```python
from build123d import *

# Parameters (mm, degrees)
PAD001_DEPTH = 12
SKETCH_W     = 24
SKETCH_H     = 12
SKETCH_R     = 1.3
PAD_DEPTH    = 2
FILLET_R     = 3
FILLET001_R  = 0.5


with BuildPart() as pad001:
    # Sketch001 → Pad001 (new body, symmetric)
    with BuildSketch(Plane.YZ):
        Polygon((0, 0), (0, 6), (2, 6), (2, 8), (0, 8), (0, 9), (7, 9), (7, 0), align=None)
    extrude(amount=PAD001_DEPTH, both=True)


with BuildPart() as fillet001:
    # Sketch → Pad (new body)
    with BuildSketch(Plane.XY):
        with Locations((0, 6)):
            Rectangle(SKETCH_W, SKETCH_H)
        with Locations((-8, 9.5)):
            Circle(SKETCH_R, mode=Mode.SUBTRACT)
        with Locations((0, 9.5)):
            Circle(SKETCH_R, mode=Mode.SUBTRACT)
        with Locations((8, 9.5)):
            Circle(SKETCH_R, mode=Mode.SUBTRACT)
    extrude(amount=-PAD_DEPTH)

    # Fusion: union Pad001
    add(pad001.part)

    # Fillet
    fillet_edges = [fillet001.edges().sort_by_distance(p)[0] for p in [
        (0, 7, 9),
    ]]
    fillet(fillet_edges, radius=FILLET_R)

    # Fillet001
    fillet001_edges = [fillet001.edges().sort_by_distance(p)[0] for p in [
        (0, 7, 0),
    ]]
    fillet(fillet001_edges, radius=FILLET001_R)


solid = fillet001.part
```
Here's how the part is built. I have some questions about the finished solid (model axes, mm). A direction names the side the tool comes from. Give positions to 0.01 mm unless a question says otherwise; leave off trailing zeros. Loops run counter-clockwise (first coordinate to the right, second up) from the corner with the lowest first, then second, coordinate; pieces in that order, holes last. Notation, with made-up numbers: M 88,16 L 131,16 A10 cw 131,25 Z; hole C 47.25,73.5 d5. An arc over 180 degrees is marked long. Put each result on its own line as item: value. Start each with the question number.
(1) I want a section at B-B on x = -8. Please give me the cut outline in (y, z).
(2) I want a section at A-A on y = 1. Please give me the cut outline in (x, z), then the cut area to 3 significant figures.
(3) I want a section at C-C on y = 9.5. Please give me the cut outline in (x, z), then the cut area to 3 significant figures.
(4) For faces 1 (the flat face through (0, 2, 7)), 2 (the flat face through (0.2, 0, 8.5)), 3 (the flat face through (0, 11, 0)), which set-ups out of +Z, -Z, +X, -X, +Y, -Y let a thin tool reach every point of the face, with its end or its side?
(5) I need wall thicknesses on line 1 along Z through (x, y) = (9.75, 0.5); line 2 along Y through (x, z) = (-8, -0.8); line 3 along Z through (x, y) = (7.25, 7.75). Which ranges of each line are inside material? Lowest first, please. Write a range as [from, to].
(6) If we mould it in two halves opening along Z, with no side actions, what happens to faces 4 (the flat face through (0, 1, 6)), 5 (the cylindrical face through (0.17, 6.14, 8.1)), 6 (the flat face through (12, 5, 2))? For each: +Z half, -Z half, draft (parallel to the pull), parting line (faces both ways), or undercut.
(7) Will these pins go through, and if not, where does the flat tip stop? pin 1 Ø1.6 at (x, z) = (5.5, 2) entering from +Y; pin 2 Ø1.6 at (x, z) = (1, 7) entering from -Y; pin 3 Ø2 at (x, y) = (3, 9) entering from +Z.
(8) I want a section at D-D on x = 10. Please give me the cut outline in (y, z), then the cut area to 3 significant figures.
Answer block:
1. outline: M 0,-2 L 8.2,-2 L 8.2,0 L 7.5,0 A0.5 cw 7,0.5 L 7,6 A3 ccw 4,9 L 0,9 L 0,8 L 2,8 L 2,6 L 0,6 Z; M 10.8,-2 L 12,-2 L 12,0 L 10.8,0 Z
2. outline: M -12,-2 L 12,-2 L 12,6 L -12,6 Z; M -12,8 L 12,8 L 12,9 L -12,9 Z
2. area: 216 mm^2
3. outline: M -12,-2 L -9.3,-2 L -9.3,0 L -12,0 Z; M -6.7,-2 L -1.3,-2 L -1.3,0 L -6.7,0 Z; M 1.3,-2 L 6.7,-2 L 6.7,0 L 1.3,0 Z; M 9.3,-2 L 12,-2 L 12,0 L 9.3,0 Z
3. area: 32.4 mm^2
4. face 1: +X, -X, -Y
4. face 2: +Z, -Z, +X, -X, -Y
4. face 3: +Z, +X, -X, +Y
5. line 1: [-2, 6], [8, 9]
5. line 2: [0, 8.2], [10.8, 12]
5. line 3: [-2, 0]
6. face 4: undercut
6. face 5: +Z half
6. face 6: draft
7. pin 1: y = 7
7. pin 2: y = 2
7. pin 3: z = 0
8. outline: M 0,-2 L 12,-2 L 12,0 L 7.5,0 A0.5 cw 7,0.5 L 7,6 A3 ccw 4,9 L 0,9 L 0,8 L 2,8 L 2,6 L 0,6 Z
8. area: 81.1 mm^2
